Could you check a few things on this model? Use its own coordinates, in mm. Face numbers are marked on the shaded views. A direction names the side the tool comes from. Give positions to 0.01 mm unless a question says otherwise; leave off trailing zeros. Write each loop counter-clockwise with the first axis right and the second up, starting at its lowest first coordinate (ties: lowest second). Pieces come first, ordered by that corner, then holes. Notation, with made-up numbers: (86, 15) - (100, 15) arc R17 cw to (100, 34) - close; hole circle Ø7 at (24.25, 85.25). An arc over 180 degrees is marked (long way). Answer in a Markdown table with one row per item.
from build123d import *
from build123d.topology import SkipClean

# Parameters (mm, degrees)
SKETCH1_R           = 30
SKETCH1_R_2         = 2.1
BOSS_EXTRUDE1_DEPTH = 5
CUT_EXTRUDE2_DEPTH  = 2
BOSS_EXTRUDE5_DEPTH = 15
SKETCH8_R           = 3
CUT_EXTRUDE3_DEPTH  = 65.101482042
CUT_EXTRUDE4_REACH  = 50.877
CUT_EXTRUDE5_REACH  = 61.237
BOSS_EXTRUDE8_DEPTH = 3
CUT_EXTRUDE8_START  = -2
CUT_EXTRUDE8_DEPTH  = 2
SKETCH14_R          = 2
BOSS_EXTRUDE9_DEPTH = 4


with BuildPart() as part:
    # Sketch1 → Boss-Extrude1 (new body)
    with BuildSketch(Plane(origin=(0, 0, 0), x_dir=(1, 0, 0), z_dir=(0, 1, 0))):
        with Locations(Location((0, 0, 0), (0, 0, 270))):
            Circle(SKETCH1_R)
        with Locations(Location((0, 15, 0), (0, 0, 270))):
            Circle(SKETCH1_R_2, mode=Mode.SUBTRACT)
        with Locations(Location((12.990381057, -7.5, 0), (0, 0, 270))):
            Circle(SKETCH1_R_2, mode=Mode.SUBTRACT)
        with Locations(Location((-12.990381057, -7.5, 0), (0, 0, 270))):
            Circle(SKETCH1_R_2, mode=Mode.SUBTRACT)
    extrude(amount=BOSS_EXTRUDE1_DEPTH)

    # Sketch7 → Cut-Extrude2 (cut)
    with BuildSketch(Plane(origin=(0, 5, 0), x_dir=(1, 0, 0), z_dir=(0, 1, 0))):
        Polygon((0, 19.156921938), (-3.6, 17.078460969), (-3.6, 12.921539031), (0, 10.843078062), (3.6, 12.921539031), (3.6, 17.078460969), align=None)
        Polygon((12.990381057, -3.343078062), (9.390381057, -5.421539031), (9.390381057, -9.578460969), (12.990381057, -11.656921938), (16.590381057, -9.578460969), (16.590381057, -5.421539031), align=None)
        Polygon((-12.990381057, -3.343078062), (-16.590381057, -5.421539031), (-16.590381057, -9.578460969), (-12.990381057, -11.656921938), (-9.390381057, -9.578460969), (-9.390381057, -5.421539031), align=None)
    extrude(amount=-CUT_EXTRUDE2_DEPTH, mode=Mode.SUBTRACT)

    # Sketch2 → Boss-Extrude5 (add)
    with BuildSketch(Plane(origin=(0, 5, 0), x_dir=(1, 0, 0), z_dir=(0, 1, 0))):
        with BuildLine():
            Line((23, -19.261360284), (23, 19.261360284))
            ThreePointArc((23, 19.261360284), (20.18526342, 22.193583322), (17, 24.718414189))
            Line((17, 24.718414189), (17, -24.718414189))
            ThreePointArc((17, -24.718414189), (20.18526342, -22.193583322), (23, -19.261360284))
        make_face()
        with BuildLine():
            Line((9, -28.618176043), (9, 28.618176043))
            ThreePointArc((9, 28.618176043), (6.798137481, 29.219605178), (4.556921938, 29.651888008))
            Line((4.556921938, 29.651888008), (4.556921938, 13.6966679))
            Line((4.556921938, 13.6966679), (3, 11))
            Line((3, 11), (3, -29.849623113))
            ThreePointArc((3, -29.849623113), (6.031510215, -29.387427321), (9, -28.618176043))
        make_face()
    boss_extrude5 = extrude(amount=BOSS_EXTRUDE5_DEPTH)

    # Sketch8 → Cut-Extrude3 (cut, through all)
    with BuildSketch(Plane(origin=(23, 0, 0), x_dir=(0, 0, -1), z_dir=(1, 0, 0))):
        with Locations((0, 13)):
            Circle(SKETCH8_R)
    cut_extrude3 = extrude(amount=-CUT_EXTRUDE3_DEPTH, mode=Mode.SUBTRACT)

    # Sketch9 → Cut-Extrude4 (cut, up to next)
    with BuildSketch(Plane.ZY.offset(-3), mode=Mode.PRIVATE) as cut_extrude4_sk1:
        Polygon((-29.651888008, 20), (-29.651888008, 5.105559505), (-11, 15.062739712), (-11, 20), (-13.6966679, 20), align=None)
    cut_extrude4_tool1 = extrude(cut_extrude4_sk1.sketch, amount=-CUT_EXTRUDE4_REACH, mode=Mode.PRIVATE) & part.part
    # Sketch9 → Cut-Extrude4 (cut, up to next)
    with BuildSketch(Plane.ZY.offset(-3), mode=Mode.PRIVATE) as cut_extrude4_sk2:
        with BuildLine():
            Line((-11, 20), (-11, 15.062739712))
            Line((-11, 15.062739712), (-3.29656778, 19.175163226))
            ThreePointArc((-3.29656778, 19.175163226), (-1.699096439, 19.790660593), (0, 20))
            Line((0, 20), (-11, 20))
        make_face()
    cut_extrude4_tool2 = extrude(cut_extrude4_sk2.sketch, amount=-CUT_EXTRUDE4_REACH, mode=Mode.PRIVATE) & part.part
    # Sketch9 → Cut-Extrude4 (cut, up to next)
    with BuildSketch(Plane.ZY.offset(-3), mode=Mode.PRIVATE) as cut_extrude4_sk3:
        with BuildLine():
            Line((29.849623113, 20), (0, 20))
            ThreePointArc((0, 20), (1.699096439, 19.790660593), (3.29656778, 19.175163226))
            Line((3.29656778, 19.175163226), (29.849623113, 5))
            Line((29.849623113, 5), (29.849623113, 20))
        make_face()
    cut_extrude4_tool3 = extrude(cut_extrude4_sk3.sketch, amount=-CUT_EXTRUDE4_REACH, mode=Mode.PRIVATE) & part.part
    cut_extrude4_1 = cut_extrude4_tool1.solids().sort_by_distance((3, 14.625463, -21.886747))[0]
    add(cut_extrude4_1, mode=Mode.SUBTRACT)
    cut_extrude4_2 = cut_extrude4_tool2.solids().sort_by_distance((3, 18.370055, -7.850815))[0]
    add(cut_extrude4_2, mode=Mode.SUBTRACT)
    cut_extrude4_3 = cut_extrude4_tool3.solids().sort_by_distance((3, 15.00565, 20.461626))[0]
    add(cut_extrude4_3, mode=Mode.SUBTRACT)
    cut_extrude4 = cut_extrude4_1 + cut_extrude4_2 + cut_extrude4_3  # Cut-Extrude4 as one shape, for the pattern or mirror that repeats it

    # Sketch10 → Cut-Extrude5 (cut, up to next)
    with BuildSketch(Plane.ZY.offset(-17), mode=Mode.PRIVATE) as cut_extrude5_sk1:
        with BuildLine():
            Line((-24.718414189, 20), (-24.718414189, 5))
            Line((-24.718414189, 5), (-3.870106441, 18.832861745))
            ThreePointArc((-3.870106441, 18.832861745), (-2.021134326, 19.701866608), (-3.6e-08, 20))
            Line((-3.6e-08, 20), (-24.718414189, 20))
        make_face()
    cut_extrude5_tool1 = extrude(cut_extrude5_sk1.sketch, amount=-CUT_EXTRUDE5_REACH, mode=Mode.PRIVATE) & part.part
    # Sketch10 → Cut-Extrude5 (cut, up to next)
    with BuildSketch(Plane.ZY.offset(-17), mode=Mode.PRIVATE) as cut_extrude5_sk2:
        with BuildLine():
            Line((3.870106441, 18.832861745), (24.718414189, 5))
            Line((24.718414189, 5), (24.718414189, 20))
            Line((24.718414189, 20), (-3.6e-08, 20))
            ThreePointArc((-3.6e-08, 20), (2.021134291, 19.701866619), (3.870106441, 18.832861745))
        make_face()
    cut_extrude5_tool2 = extrude(cut_extrude5_sk2.sketch, amount=-CUT_EXTRUDE5_REACH, mode=Mode.PRIVATE) & part.part
    cut_extrude5_1 = cut_extrude5_tool1.solids().sort_by_distance((17, 15.01191, -17.14476))[0]
    add(cut_extrude5_1, mode=Mode.SUBTRACT)
    cut_extrude5_2 = cut_extrude5_tool2.solids().sort_by_distance((17, 15.01191, 17.14476))[0]
    add(cut_extrude5_2, mode=Mode.SUBTRACT)
    cut_extrude5 = cut_extrude5_1 + cut_extrude5_2  # Cut-Extrude5 as one shape, for the pattern or mirror that repeats it

    # Mirror1: Boss-Extrude5, Cut-Extrude3, Cut-Extrude4, Cut-Extrude5 across plane
    with SkipClean():  # the faces are left unmerged after this step: merging them gives an invalid solid
        add(boss_extrude5.mirror(Plane.ZY))
        add(cut_extrude3.mirror(Plane.ZY), mode=Mode.SUBTRACT)
        add(cut_extrude4.mirror(Plane.ZY), mode=Mode.SUBTRACT)
        add(cut_extrude5.mirror(Plane.ZY), mode=Mode.SUBTRACT)

    # Sketch13 → Boss-Extrude8 (add)
    with SkipClean():  # the faces are left unmerged after this step: merging them gives an invalid solid
        with BuildSketch(Plane.XZ):
            with BuildLine():
                ThreePointArc((12.385089192, -31.30324211), (15.3125, -31.472644372), (16.98597293, -29.064757431))
                Line((16.98597293, -29.064757431), (17.437516579, -24.411739298))
                ThreePointArc((17.437516579, -24.411739298), (13.125, -26.976552319), (8.445332472, -28.786739298))
                Line((8.445332472, -28.786739298), (12.385089192, -31.30324211))
            make_face()
        boss_extrude8 = extrude(amount=-BOSS_EXTRUDE8_DEPTH)

    # Sketch15 → Cut-Extrude8 (cut)
    with SkipClean():  # the faces are left unmerged after this step: merging them gives an invalid solid
        with BuildSketch(Plane(origin=(0, 5, 0), x_dir=(1, 0, 0), z_dir=(0, 1, 0)).offset(CUT_EXTRUDE8_START)):
            with BuildLine():
                ThreePointArc((15.036417377, 25.959702472), (13.125, 26.976552319), (11.145223248, 27.852899288))
                ThreePointArc((11.145223248, 27.852899288), (12.6875, 26.077333908), (15.036417377, 25.959702472))
            make_face()
            with BuildLine():
                ThreePointArc((17, 28.77498914), (13.533272165, 31.738460943), (11.145223248, 27.852899288))
                ThreePointArc((11.145223248, 27.852899288), (13.125, 26.976552319), (15.036417377, 25.959702472))
                ThreePointArc((15.036417377, 25.959702472), (16.460614977, 27.058779964), (17, 28.77498914))
            make_face()
        cut_extrude8 = extrude(amount=CUT_EXTRUDE8_DEPTH, mode=Mode.SUBTRACT)

    # Sketch14 → Boss-Extrude9 (add)
    with SkipClean():  # the faces are left unmerged after this step: merging them gives an invalid solid
        with BuildSketch(Plane(origin=(0, 3, 0), x_dir=(1, 0, 0), z_dir=(0, 1, 0))):
            with Locations(Location((14, 28.77498914, 0), (0, 0, 90))):
                Circle(SKETCH14_R)
        boss_extrude9 = extrude(amount=BOSS_EXTRUDE9_DEPTH)

    # Mirror2: Boss-Extrude8, Cut-Extrude8, Boss-Extrude9 across plane
    with SkipClean():  # the faces are left unmerged after this step: merging them gives an invalid solid
        add(boss_extrude8.mirror(Plane.ZY))
        add(cut_extrude8.mirror(Plane.ZY), mode=Mode.SUBTRACT)
        add(boss_extrude9.mirror(Plane.ZY))


solid = part.part
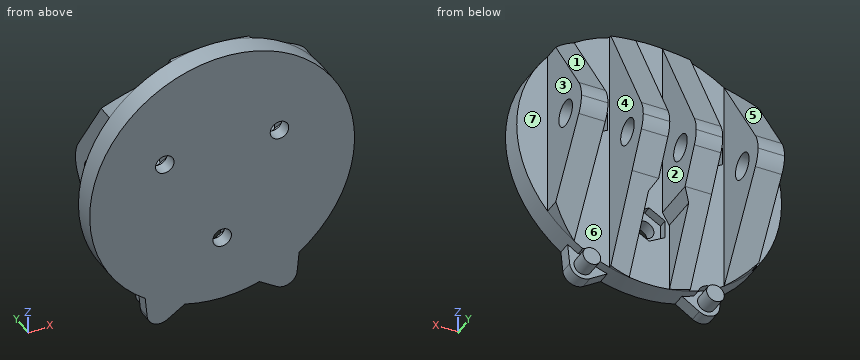
1) Imagine slicing it at A-A (y = 1.75). List the corners of the cut face in (x, z) for me, then the cut area to 3 significant figures.
Check values:
| item | result |
|---|---|
| outline | (-17.44, -24.41) - (-16.99, -29.06) arc R3 ccw to (-12.39, -31.3) - (-8.45, -28.79) arc R30 ccw to (8.45, -28.79) - (12.39, -31.3) arc R3 ccw to (16.99, -29.06) - (17.44, -24.41) arc R30 ccw (long way) to start; hole circle Ø4.2 at (-12.99, 7.5); hole circle Ø4.2 at (0, -15); hole circle Ø4.2 at (12.99, 7.5) |
| area | 2,850 mm2 |
2) If I drill on line 1 (X direction, y = 5.5, z = 7); line 2 (X direction, y = 6, z = -19); line 3 (Z direction, x = 0, y = 1.25), over which ranges is the centre line in solid material (lowest first)?
Check values:
| item | result |
|---|---|
| line 1 | x = -23 to -17, -9 to -3, 3 to 9, 17 to 23 |
| line 2 | x = -23 to -17, -9 to -4.56, 4.56 to 9, 17 to 23 |
| line 3 | z = -30 to -17.1, -12.9 to 30 |
3) Will these pins go through, and if not, where does the flat tip stop? P1, Ø1, axis at x = -12.5, z = -10.5, coming from the -Y side; P2, Ø10, axis at y = 11, z = -10, coming from the -X side; P3, Ø12, axis at y = 17.5, z = 5, coming from the +X side; P4, Ø5.5, axis at x = -26, z = -3, coming from the +Y side.
Check values:
| item | result |
|---|---|
| P1 | stops at y = 0 |
| P2 | stops at x = -23 |
| P3 | stops at x = 23 |
| P4 | stops at y = 5 |
4) We'd pull the mould along X, two halves only. Please class the marked faces 1, 2, 3 and 4: +X half, -X half, draft (parallel to the pull), parting line (faces both ways), or undercut.
Check values:
| item | result |
|---|---|
| face 1 | draft |
| face 2 | undercut |
| face 3 | +X half |
| face 4 | undercut |
5) Imagine slicing it at D-D (x = -14). List the corners of the cut face in (y, z) for me, then the cut area to 3 significant figures.
Check values:
| item | result |
|---|---|
| outline | (0, -31.77) - (3, -31.77) - (3, -30.77) - (7, -30.77) - (7, -26.77) - (3, -26.77) - (3, -25.77) - (5, -25.77) - (5, 3.93) - (3, 3.93) - (3, 5.66) - (0, 5.66) - close; (0, 9.34) - (3, 9.34) - (3, 11.07) - (5, 11.07) - (5, 26.53) - (0, 26.53) - close |
| area | 270 mm2 |
6) Imagine slicing it at B-B (x = -21.5). List the corners of the cut face in (y, z) for me, then the cut area to 3 significant figures.
Check values:
| item | result |
|---|---|
| outline | (0, -20.92) - (7.52, -20.92) - (18.83, -3.87) arc R7 ccw to (18.83, 3.87) - (7.52, 20.92) - (0, 20.92) - close; hole circle Ø6 at (13, 0) |
| area | 573 mm2 |
7) Imagine slicing it at C-C (z = -15). List the corners of the cut face in (x, y) for me.
Check values:
| item | result |
|---|---|
| outline | (-25.98, 0) - (-2.1, 0) - (-2.1, 3) - (-3.6, 3) - (-3.6, 5) - (-4.56, 5) - (-4.56, 12.93) - (-9, 12.93) - (-9, 5) - (-17, 5) - (-17, 11.45) - (-23, 11.45) - (-23, 5) - (-25.98, 5) - close; (2.1, 0) - (25.98, 0) - (25.98, 5) - (23, 5) - (23, 11.45) - (17, 11.45) - (17, 5) - (9, 5) - (9, 12.93) - (4.56, 12.93) - (4.56, 5) - (3.6, 5) - (3.6, 3) - (2.1, 3) - close |
8) On a 3-axis mill with a long thin cutter (end or side, diameter ignored), from which of +Z, -Z, +X, -X, +Y, -Y can I reach the whole of each face in a straight line? I mean the marked faces 5, 6 and 7. Say none if no direction works.
Check values:
| item | result |
|---|---|
| face 5 | +Z, -X, +Y |
| face 6 | +Z, +Y |
| face 7 | +Z, -Z, +X, +Y |
